Geometry check sheet. Reference: the model listing, model coordinates, mm. Face numbers are marked on the shaded views. A direction names the side the tool comes from. Coordinates: 2 decimals unless noted, no trailing zeros. Loops run counter-clockwise (first coordinate to the right, second up) from the corner with the lowest first, then second, coordinate; pieces in that order, holes last.
from build123d import *

# Parameters (mm, degrees)
F0_R     = 10
F1_DEPTH = 20
F3_DEPTH = 8
F4_R     = 3.1
F5_DEPTH = 7
F6_R     = 1.4
F7_DEPTH = 12.5


with BuildPart() as f1:
    # F0 (on Front) → F1 (new body)
    with BuildSketch(Plane.XZ):
        Circle(F0_R)
    extrude(amount=F1_DEPTH)

    # F2 (on face) → F3 (cut)
    with BuildSketch(Plane.XZ.offset(20)):
        with BuildLine():
            Line((1.75, -2.12132), (1.75, 2.12132))
            ThreePointArc((1.75, 2.12132), (0, 2.75), (-1.75, 2.12132))
            Line((-1.75, 2.12132), (-1.75, -2.12132))
            ThreePointArc((-1.75, -2.12132), (0, -2.75), (1.75, -2.12132))
        make_face()
    extrude(amount=-F3_DEPTH, mode=Mode.SUBTRACT)

    # F4 (on face) → F5 (cut)
    with BuildSketch(Plane(origin=(0, 0, 0), x_dir=(-1, 0, 0), z_dir=(0, 1, 0))):
        Circle(F4_R)
    extrude(amount=-F5_DEPTH, mode=Mode.SUBTRACT)

    # F6 (on Right) → F7 (cut, symmetric)
    with BuildSketch(Plane.YZ):
        with Locations((-3.5, 0)):
            Circle(F6_R)
        with Locations((-16.5, 0)):
            Circle(F6_R)
    extrude(amount=F7_DEPTH, both=True, mode=Mode.SUBTRACT)


solid = f1.part
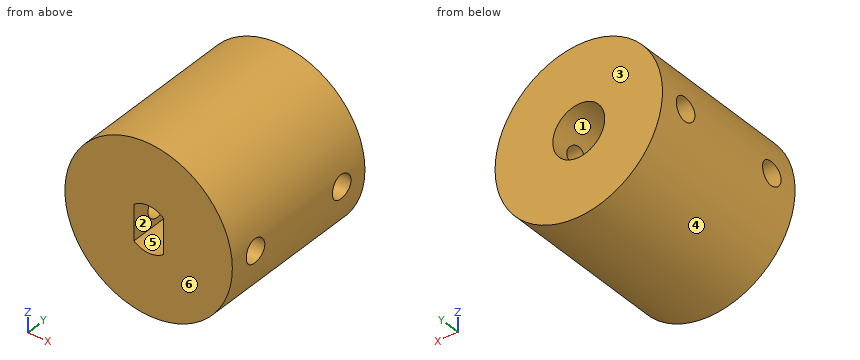
1) Section check A-A on z = 0. Record the cut outline in (x, y), and give its area (3 significant figures).
Data:
outline: (-10, -20) - (-1.75, -20) - (-1.75, -17.9) - (-10, -17.9) - close; (-10, -15.1) - (-1.75, -15.1) - (-1.75, -12) - (1.75, -12) - (1.75, -15.1) - (10, -15.1) - (10, -4.9) - (3.1, -4.9) - (3.1, -7) - (-3.1, -7) - (-3.1, -4.9) - (-10, -4.9) - close; (-10, -2.1) - (-3.1, -2.1) - (-3.1, 0) - (-10, 0) - close; (1.75, -20) - (10, -20) - (10, -17.9) - (1.75, -17.9) - close; (3.1, -2.1) - (10, -2.1) - (10, 0) - (3.1, 0) - close
area: 244 mm2
2) Section check D-D on x = 0. Record the cut outline in (y, z), and give its area (3 significant figures).
Data:
outline: (-20, -10) - (0, -10) - (0, -3.1) - (-7, -3.1) - (-7, 3.1) - (0, 3.1) - (0, 10) - (-20, 10) - (-20, 2.75) - (-12, 2.75) - (-12, -2.75) - (-20, -2.75) - close
area: 313 mm2
3) Depth check by flat-ended pin: pin 1 (3 mm diameter, centred on y = -3.5, z = -0.5, fed in from -X); pin 2 (12 mm diameter, centred on x = 7.5, y = -6.5, fed in from -Z); pin 3 (4 mm diameter, centred on y = -10, z = 6.5, fed in from -X); pin 4 (1.5 mm diameter, centred on x = 5.5, y = -6, fed in from +Z). Enter the tip coordinate at first touch or a pass-through.
Data:
pin 1: stops at x = -10
pin 2: stops at z = -9.89
pin 3: stops at x = -8.93
pin 4: stops at z = 8.8
4) Section check B-B on y = -3.5. Record the cut outline in (x, z).
Data:
outline: (-9.9, -1.4) arc R10 ccw to (9.9, -1.4) - (2.77, -1.4) arc R3.1 cw to (-2.77, -1.4) - close; (-9.9, 1.4) - (-2.77, 1.4) arc R3.1 cw to (2.77, 1.4) - (9.9, 1.4) arc R10 ccw to start
5) Mould release check, pull along X, two halves, no side actions. Record for the marked faces 1, 2, 3 and 4: +X half, -X half, draft (parallel to the pull), parting line (faces both ways), or undercut.
Data:
face 1: undercut
face 2: undercut
face 3: draft
face 4: parting line
6) Access from +Z, -Z, +X, -X, +Y, -Y to the whole of each face (thin tool, end or side, straight path). Record for the marked faces 5 and 6.
Data:
face 5: -Y
face 6: +Z, -Z, +X, -X, -Y
7) Section check C-C on x = 6. Record the cut outline in (y, z).
Data:
outline: (-20, -8) - (0, -8) - (0, 8) - (-20, 8) - close; hole circle Ø2.8 at (-16.5, 0); hole circle Ø2.8 at (-3.5, 0)
8) Material ranges on probe 1 along Y at (x, z) = (-5.25, 0); probe 2 along X at (y, z) = (-2, 0), recorded low to high.
Data:
probe 1: y = -20 to -17.9, -15.1 to -4.9, -2.1 to 0
probe 2: x = -10 to -3.1, 3.1 to 10
